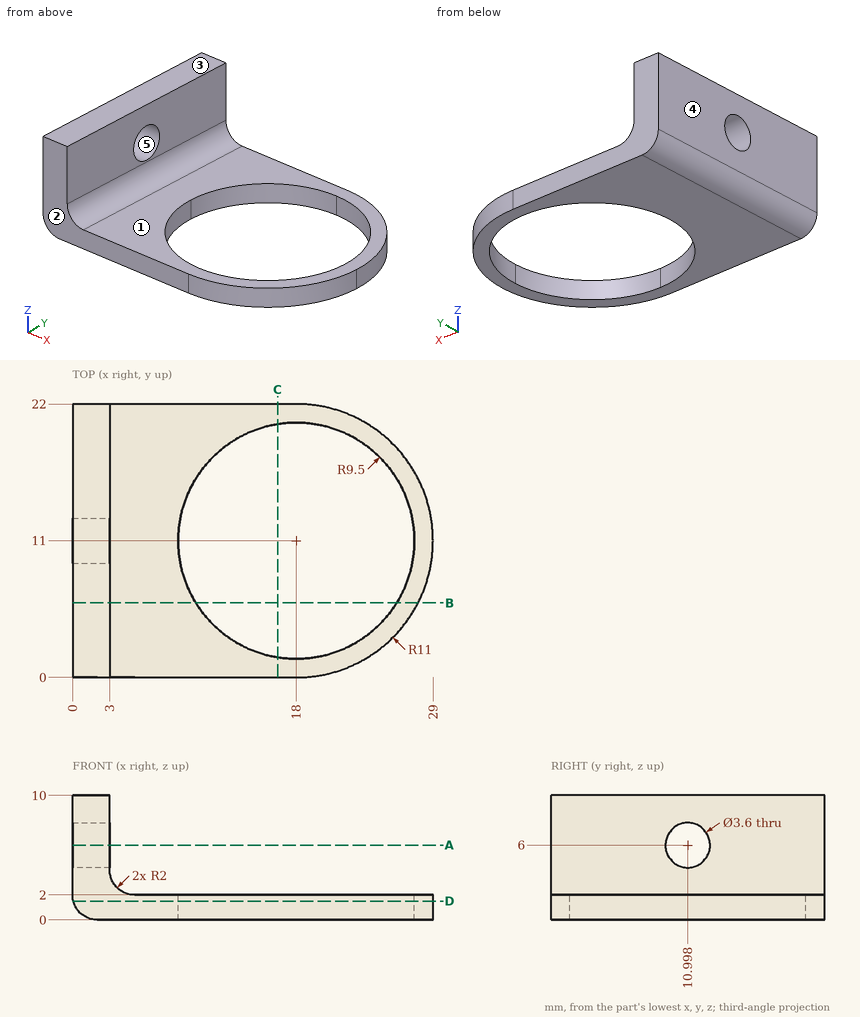
The drawing under review shows one solid part. Ordinate dimensions are in mm from its lowest x, y, z. A direction names the side the tool comes from. Give positions to 0.01 mm unless a question says otherwise; leave off trailing zeros. Write each loop counter-clockwise with the first axis right and the second up, starting at its lowest first coordinate (ties: lowest second). Pieces come first, ordered by that corner, then holes. Notation, with made-up numbers: (-11.5, -15.75) -> (14.5, -15.75) arc R13 ccw to (14.5, -1.75) -> close; hole circle Ø4 at (12.5, 82.25). An arc over 180 degrees is marked (long way). Answer in a Markdown table with one row per item.
(1) Consider section C-C (x = 16.5). State the section outline as (y, z) points.
Results:
| item | result |
|---|---|
| outline | (0, 0) -> (1.62, 0) -> (1.62, 2) -> (0, 2) -> close; (20.38, 0) -> (22, 0) -> (22, 2) -> (20.38, 2) -> close |
(2) Clearance check with flat-ended pins moving along their axes: pin 1 (10 mm diameter, centred on x = 9, y = 16.5, fed in from +Z); pin 2 (1.5 mm diameter, centred on y = 17, z = 6.5, fed in from +X); pin 3 (6.5 mm diameter, centred on x = 13, y = 15, fed in from +Z); pin 4 (3 mm diameter, centred on x = 15.5, y = 16.5, fed in from +Z). State where each tip first meets the part, or that it passes through.
Results:
| item | result |
|---|---|
| pin 1 | z = 2.27 |
| pin 2 | x = 3 |
| pin 3 | z = 2 |
| pin 4 | through |
(3) Mouldability with a two-part tool opening along Z and no side actions: class the marked faces 3, 4 and 5 as +Z half, -Z half, draft (parallel to the pull), parting line (faces both ways), or undercut.
Results:
| item | result |
|---|---|
| face 3 | +Z half |
| face 4 | draft |
| face 5 | undercut |
(4) Consider section B-B (y = 6). State the section outline as (x, z) points.
Results:
| item | result |
|---|---|
| outline | (0, 2) arc R2 ccw to (2, 0) -> (9.92, 0) -> (9.92, 2) -> (5, 2) arc R2 cw to (3, 4) -> (3, 10) -> (0, 10) -> close; (26.08, 0) -> (27.8, 0) -> (27.8, 2) -> (26.08, 2) -> close |
(5) Consider section D-D (z = 1.5). State the section outline as (x, y) points, then the cut area to 3 significant figures.
Results:
| item | result |
|---|---|
| outline | (0.06, 0) -> (18, 0) arc R11 ccw to (18, 22) -> (0.06, 22) -> close; hole circle Ø19 at (18, 11) |
| area | 301 mm2 |
(6) To check wall thickness, follow probe 1 along Y at (x, z) = (1.5, 6); probe 2 along Z at (x, y) = (27, 14.5); probe 3 along X at (y, z) = (20.75, 4.25). State the ranges of each line that lie inside material, in increasing order.
Results:
| item | result |
|---|---|
| probe 1 | 0 to 9.2, 12.8 to 22 |
| probe 2 | 0 to 2 |
| probe 3 | 0 to 3 |
(7) For the marked faces 1 and 2, list the 3-axis set-ups (+Z, -Z, +X, -X, +Y, -Y) from which the entire face can be reached by the end or side of a thin tool; tool diameter is ignored.
Results:
| item | result |
|---|---|
| face 1 | +Z, +X, +Y, -Y |
| face 2 | +Z, -Z, +X, -X, -Y |
(8) Consider section A-A (z = 6). State the section outline as (x, y) points, then the cut area to 3 significant figures.
Results:
| item | result |
|---|---|
| outline | (0, 0) -> (3, 0) -> (3, 9.2) -> (0, 9.2) -> close; (0, 12.8) -> (3, 12.8) -> (3, 22) -> (0, 22) -> close |
| area | 55.2 mm2 |
